```python
from build123d import *

# Parameters (mm, degrees)
SKETCH1_W           = 127
SKETCH1_H           = 228.6
BOSS_EXTRUDE1_DEPTH = 101.6
CUT_EXTRUDE3_DEPTH  = 188.099924105
SKETCH6_R           = 7.14375
CUT_EXTRUDE4_DEPTH  = 101.6


with BuildPart() as part:
    # Sketch1 → Boss-Extrude1 (new body)
    with BuildSketch(Plane(origin=(0, 0, 0), x_dir=(1, 0, 0), z_dir=(0, 1, 0))):
        with Locations((-25.4, -15.24)):
            Rectangle(SKETCH1_W, SKETCH1_H)
    extrude(amount=BOSS_EXTRUDE1_DEPTH)

    # Sketch3 → Cut-Extrude3 (cut, through all)
    with BuildSketch(Plane(origin=(0, 101.6, 0), x_dir=(1, 0, 0), z_dir=(0, 1, 0))):
        Polygon((34.925, 57.785), (34.925, 99.06), (-88.9, 99.06), (-88.9, -78.74), align=None)
        Polygon((38.1, -129.54), (38.1, 56.559637154), (-85.725, -79.965362846), (-85.725, -129.54), align=None)
    extrude(amount=-CUT_EXTRUDE3_DEPTH, mode=Mode.SUBTRACT)

    # Sketch6 → Cut-Extrude4 (cut)
    with BuildSketch(Plane(origin=(38.1, 0, 0), x_dir=(0, 0, -1), z_dir=(1, 0, 0))):
        with Locations((77.809818577, 76.2)):
            Circle(SKETCH6_R)
        with Locations((77.809818577, 25.4)):
            Circle(SKETCH6_R)
    extrude(amount=-CUT_EXTRUDE4_DEPTH, mode=Mode.SUBTRACT)


solid = part.part
```
Could you check a few things on this model? Use its own coordinates, in mm. A direction names the side the tool comes from. Round coordinates to 2 decimals unless told otherwise and drop trailing zeros. Order: outer loops, then holes, each group sorted by start corner. A loop starts at its lowest first (then second) coordinate and runs counter-clockwise, first axis right, second up. Notation, with made-up numbers: M 87.5,85.5 L 109.5,85.5 A27 cw 109.5,106.5 Z; hole C 31,22.25 d5. An arc over 180 degrees is marked long. One line per question, with ' | ' between items. Start each with the question number.
(1) Suppose I cut it at C-C on z = 19. List the corners of the cut face in (x, y) for me.
(2) Thinking about a two-plate mould opening in Z: for faces 1 (the face through (-85.725, 52, 104)), 2 (the face through (36.535, 25.714, -70.673)), 3 (the face through (-22.95, 51.51, 10.75)), which applies, +Z half, -Z half, draft (parallel to the pull), parting line (faces both ways), or undercut?
(3) Please list where these lines run through material, in increasing order: line 1 along X through (y, z) = (59, -72.5) (3 decimals); line 2 along X through (y, z) = (39.5, 89.5) (3 decimals); line 3 along Z through (x, y) = (26.5, 6.5).
(4) Suppose I cut it at A-A on y = 25.4. List the corners of the cut face in (x, z) for me (3 decimals).
(5) For faces 4 (the face through (-30, 0, 15)), 5 (the face through (34.925, 52, -78)), which set-ups out of +Z, -Z, +X, -X, +Y, -Y let a thin tool reach every point of the face, with its end or its side?
(6) Suppose I cut it at D-D on y = 79. List the corners of the cut face in (x, z) for me (3 decimals), then the cut area to 3 significant figures.
(7) Suppose I cut it at B-B on y = 49.5. List the corners of the cut face in (x, z) for me (3 decimals), then the cut area to 3 significant figures.
(8) For P1, Ø18.5, axis at y = 25.4, z = -77.81, coming from the -X side (3 decimals); P2, Ø8, axis at x = -1.5, y = 76.5, coming from the -Z side; P3, Ø4, axis at y = 32, z = -10, coming from the -X side; P4, Ø11.5, axis at y = 76.2, z = -77.81, coming from the +X side (1 decimal), each with a flat end and sliding along its axis, tell me the tip position at first contact or that it passes through.
Geometry results:
1) outline: M -34.72,0 L -30.43,0 L -30.43,101.6 L -34.72,101.6 Z
2) face 1: draft | face 2: undercut | face 3: +Z half
3) line 1: 34.925 to 38.1 | line 2: -88.9 to -85.725 | line 3: -48.5 to -43.77
4) outline: M -88.9,78.74 L 34.925,-57.785 L 34.925,-70.666 L 38.1,-70.666 L 38.1,-56.56 L -85.725,79.965 L -85.725,129.54 L -88.9,129.54 Z; M 34.925,-99.06 L 38.1,-99.06 L 38.1,-84.954 L 34.925,-84.954 Z
5) face 4: +Z, -Z, +X, -X, -Y | face 5: -Z, -X, +Y, -Y
6) outline: M -88.9,78.74 L 34.925,-57.785 L 34.925,-71.238 L 38.1,-71.238 L 38.1,-56.56 L -85.725,79.965 L -85.725,129.54 L -88.9,129.54 Z; M 34.925,-99.06 L 38.1,-99.06 L 38.1,-84.382 L 34.925,-84.382 Z | area: 836 mm²
7) outline: M -88.9,78.74 L 34.925,-57.785 L 34.925,-99.06 L 38.1,-99.06 L 38.1,-56.56 L -85.725,79.965 L -85.725,129.54 L -88.9,129.54 Z | area: 878 mm²
8) P1: x = 34.925 | P2: z = -22.03 | P3: x = -10.23 | P4: through
